Autodesk Inventor part; units mm, degrees
ref_plane "YZ Plane" through (0, 0, 0) normal (1, 0, 0) x (0, 1, 0)
ref_plane "XZ Plane" through (0, 0, 0) normal (0, 1, 0) x (-1, 0, 0)
ref_plane "XY Plane" through (0, 0, 0) normal (0, 0, 1) x (1, 0, 0)
sketch "Sketch1" plane through (0, 0, 0) normal (1, 0, 0) x (0, 1, 0)
  circle A0 centre (0, 0) radius 12.5 construction
  line L0 (6.25, 10.8253) -> (0, 0) construction
  line L1 (0, 0) -> (-12.5, 0) construction
  line L2 (0, 0) -> (6.25, -10.8253) construction
  line L3 (0, 12.5) -> (0, -12.5) construction
  circle A1 centre (6.25, 10.8253) radius 1.5
  circle A2 centre (6.25, -10.8253) radius 1.5
  circle A3 centre (-12.5, 0) radius 1.5
  circle A4 centre (0, 0) radius 22.5
  circle A5 centre (-100, 0) radius 25
  circle A6 centre (-100, 0) radius 21.2132 construction
  arc A7 (-94.8324, 24.4601) -> (-3.5634, 22.216) centre (-43.1562, 269.0609) ccw
  arc A8 (-3.5634, -22.216) -> (-94.8324, -24.4601) centre (-43.1562, -269.0609) ccw
  line L4 (-100, 25) -> (-100, -25) construction
  line L5 (-75, 0) -> (-125, 0) construction
  line L6 (-82.3223, 17.6777) -> (-117.6777, -17.6777) construction
  line L7 (-82.3223, -17.6777) -> (-117.6777, 17.6777) construction
  circle A9 centre (-85, 15) radius 1.5
  circle A10 centre (-85, -15) radius 1.5
  circle A11 centre (-115, -15) radius 1.5
  circle A12 centre (-115, 15) radius 1.5
  point P0 (-94.8324, -24.4601)
  point P1 (-3.5634, -22.216)
  dimension "d4" = 45
  dimension "d6" = 50
  dimension "d0" = 25
  dimension "d1" = 30
  dimension "d2" = 30
  dimension "d3" = 3
  dimension "d8" = 100
  dimension "d9" = 500
  dimension "d10" = 45
  dimension "d11" = 45
  dimension "d12" = 3
  dimension "d15" = 30
extrude "Extrusion1" add sketch "Sketch1" along normal blind 15
fillet "Fillet1" radius 2 8 edges at (15, -49.3012, 19.1365) (15, -125, 0) (15, -49.3012, -19.1365) (15, 22.5, 0) (0, -49.3012, 19.1365) (0, -125, 0) (0, -49.3012, -19.1365) (0, 22.5, 0)
properties part number "leg_demo_8"
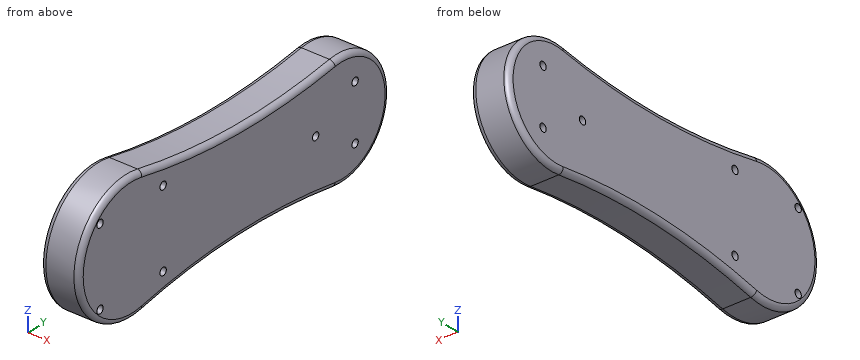
The model under review builds one solid part; all positions refer to its coordinate system, in mm. Round coordinates to 2 decimals unless told otherwise and drop trailing zeros. Write each loop counter-clockwise with the first axis right and the second up, starting at its lowest first coordinate (ties: lowest second). Pieces come first, ordered by that corner, then holes. Notation, with made-up numbers: (40.5, 36) - (51.5, 36) arc R19 cw to (51.5, 67) - close; hole circle Ø1 at (-8, -26.75). An arc over 180 degrees is marked (long way). Answer as CSV lines item,"result". Start each with the question number.
(1) We need section A-A on z = 0. State the section outline as (x, y) points, plus the area to 3 significant figures.
(2) To check wall thickness, follow line 1 (Z direction, x = 9.5, y = 6.25); line 2 (Z direction, x = 12, y = -85); line 3 (Z direction, x = 6.5, y = -12.5). State the ranges of each line that lie inside material, in increasing order.
(3) We need section B-B on x = 4. State the section outline as (y, z) points.
(4) We need section C-C on y = -85. Give the number of separate pieces and of enclosed holes in the cut face, plus the area to 3 significant figures.
(5) For pin 1 Ø3 at (x, z) = (13, -12) entering from +Y; pin 2 Ø2.5 at (y, z) = (-85, -15) entering from +X; pin 3 Ø1 at (x, z) = (12.5, -8) entering from -Y; pin 4 Ø3.5 at (y, z) = (-115, 15) entering from -X, all flat-tipped, find the tip position at first contact; note any pin that passes through.
Worked answers:
1,outline,"(0, -123) arc R2 ccw to (2, -125) - (13, -125) arc R2 ccw to (15, -123) - (15, -14) - (0, -14) - close; (0, -11) - (15, -11) - (15, 20.5) arc R2 ccw to (13, 22.5) - (2, 22.5) arc R2 ccw to (0, 20.5) - close"
1,area,"2,160 mm²"
2,line 1,"-21.61 to -12.33, -9.33 to 9.33, 12.33 to 21.61"
2,line 2,"-22.59 to -16.5, -13.5 to 13.5, 16.5 to 22.59"
2,line 3,"-20.95 to -1.5, 1.5 to 20.95"
3,outline,"(-94.83, -24.46) arc R250 cw to (-3.56, -22.22) arc R22.5 ccw (long way) to (-3.56, 22.22) arc R250 cw to (-94.83, 24.46) arc R25 ccw (long way) to start; hole circle Ø3 at (-115, -15); hole circle Ø3 at (-115, 15); hole circle Ø3 at (-85, -15); hole circle Ø3 at (-85, 15); hole circle Ø3 at (-12.5, 0); hole circle Ø3 at (6.25, -10.83); hole circle Ø3 at (6.25, 10.83)"
4,separate pieces,"3"
4,enclosed holes,"0"
4,area,"584 mm²"
5,pin 1,"y = 19.9"
5,pin 2,"through"
5,pin 3,"y = -123.85"
5,pin 4,"x = 0"
